Build history of the part. All positions in model axes, mm. Coordinates: 2 decimals unless noted, no trailing zeros. Loops run counter-clockwise (first coordinate to the right, second up) from the corner with the lowest first, then second, coordinate; pieces in that order, holes last. Notation, with made-up numbers: (15, 26) -> (60, 26) arc R19 cw to (60, 44) -> close; hole circle Ø11 at (76, 35). An arc over 180 degrees is marked (long way). One line per item, written item: value. Start each with the question number.
```python
from build123d import *

# Parameters (mm, degrees)
F0_R     = 23.368
F1_DEPTH = 1.0583333333
F0_R_2   = 29.0195
F0_R_3   = 25.8445
F2_R     = 29.0195
F2_R_2   = 23.368
F3_DEPTH = 1.0583333333
F4_R     = 29.0195
F4_R_2   = 25.8445
F4_R_3   = 23.368
F5_DEPTH = 1.0583333333
F6_R     = 0.508


with BuildPart() as f1:
    # F0 (on Top) → F1 (new body)
    with BuildSketch(Plane.XY):
        Circle(F0_R)
    extrude(amount=F1_DEPTH)



with BuildPart() as f1b:
    # F0 (on Top) → F1, piece 2 (new body)
    with BuildSketch(Plane.XY):
        Circle(F0_R_2)
        Circle(F0_R_3, mode=Mode.SUBTRACT)
    extrude(amount=F1_DEPTH)


with BuildPart() as f1_1:
    add(f1.part)

    add(f1b.part)  # F3 merges F1b
    # F2 (on face) → F3 (join)
    with BuildSketch(Plane(origin=(0, 0, 0), x_dir=(1, 0, 0), z_dir=(0, 0, -1))):
        Circle(F2_R)
        Circle(F2_R_2, mode=Mode.SUBTRACT)
        Circle(F2_R_2)
    extrude(amount=F3_DEPTH)

    # F4 (on face) → F5 (join)
    with BuildSketch(Plane(origin=(0, 0, -1.0583333333), x_dir=(1, 0, 0), z_dir=(0, 0, -1))):
        Circle(F4_R)
        Circle(F4_R_2, mode=Mode.SUBTRACT)
        Circle(F4_R_3)
    extrude(amount=F5_DEPTH)

    # F6
    f6_edges = [f1_1.edges().sort_by_distance(p)[0] for p in [
        (-29.0195, 0, -2.116667),
        (-29.0195, 0, 1.058333),
    ]]
    fillet(f6_edges, radius=F6_R)


solid = f1_1.part
```
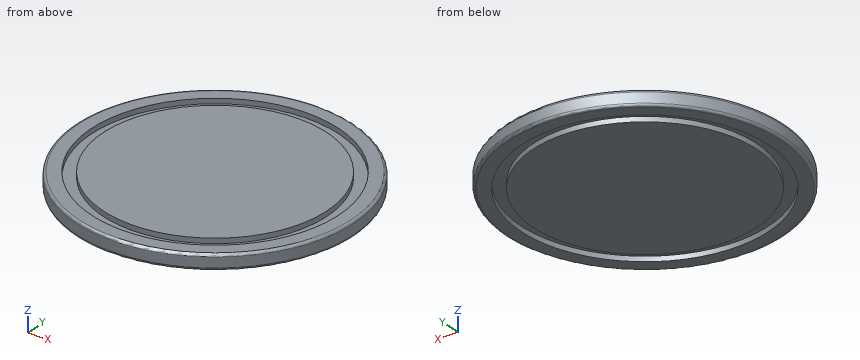
Item 1: Band-saw the part on A-A, the plane y = 0. List the corners of the cut face in (x, z).
Item 2: Probe probe 1 along X at (y, z) = (0, -1.65); probe 2 along Y at (x, z) = (3, -1.45). List the from-to ranges inside material, lowest first.
Item 3: Drop a flat-ended pin along its axis: pin 1 Ø1 at (y, z) = (-11.5, 0) entering from -X. Give the stop position or say it passes through.
Worked out:
1. outline: (-29.02, -1.61) arc R0.51 ccw to (-28.51, -2.12) -> (-25.84, -2.12) -> (-25.84, -1.06) -> (-23.37, -1.06) -> (-23.37, -2.12) -> (23.37, -2.12) -> (23.37, -1.06) -> (25.84, -1.06) -> (25.84, -2.12) -> (28.51, -2.12) arc R0.51 ccw to (29.02, -1.61) -> (29.02, 0.55) arc R0.51 ccw to (28.51, 1.06) -> (25.84, 1.06) -> (25.84, 0) -> (23.37, 0) -> (23.37, 1.06) -> (-23.37, 1.06) -> (-23.37, 0) -> (-25.84, 0) -> (-25.84, 1.06) -> (-28.51, 1.06) arc R0.51 ccw to (-29.02, 0.55) -> close
2. probe 1: x = -29.02 to -25.84, -23.37 to 23.37, 25.84 to 29.02
2. probe 2: y = -28.86 to -25.67, -23.17 to 23.17, 25.67 to 28.86
3. pin 1: stops at x = -26.85
